Source: CAD feature listing. Evaluate the final solid. Frame: model axes, mm. Round coordinates to 2 decimals unless told otherwise and drop trailing zeros. Loops run counter-clockwise (first coordinate to the right, second up) from the corner with the lowest first, then second, coordinate; pieces in that order, holes last. Notation, with made-up numbers: M 25,42 L 39,42 A22 cw 39,54 Z; hole C -22.75,76.25 d9. An arc over 180 degrees is marked long. Answer as a JSON object with one key per item and string values.
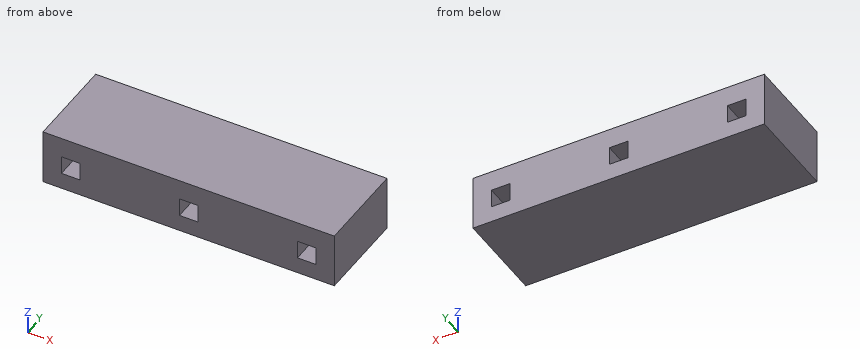
from build123d import *

# Parameters (mm, degrees)
SKETCH1_W           = 7.9
SKETCH1_H           = 1.5
SKETCH1_W_2         = 0.5
SKETCH1_H_2         = 0.5
BOSS_EXTRUDE1_DEPTH = 2.5


with BuildPart() as part:
    # Sketch1 → Boss-Extrude1 (new body)
    with BuildSketch(Plane(origin=(0, 0, 0), x_dir=(1, 0, 0), z_dir=(0, 1, 0))):
        with Locations((2.505127678, 0.264314746)):
            Rectangle(SKETCH1_W, SKETCH1_H)
        with Locations((-0.694872322, 0.316232633)):
            Rectangle(SKETCH1_W_2, SKETCH1_H_2, mode=Mode.SUBTRACT)
        with Locations((5.705127678, 0.319368521)):
            Rectangle(SKETCH1_W_2, SKETCH1_H_2, mode=Mode.SUBTRACT)
        with Locations((2.505127678, 0.311937798)):
            Rectangle(SKETCH1_W_2, SKETCH1_H_2, mode=Mode.SUBTRACT)
    extrude(amount=BOSS_EXTRUDE1_DEPTH)


solid = part.part
Item 1: Section B-B on y = 0.5. Return the cut outline in (x, z).
Answer sheet:
{"outline": "M -1.44,-1.01 L 6.46,-1.01 L 6.46,0.49 L -1.44,0.49 Z; hole M -0.94,-0.57 L -0.44,-0.57 L -0.44,-0.07 L -0.94,-0.07 Z; hole M 2.26,-0.56 L 2.76,-0.56 L 2.76,-0.06 L 2.26,-0.06 Z; hole M 5.46,-0.57 L 5.96,-0.57 L 5.96,-0.07 L 5.46,-0.07 Z"}
Item 2: Section A-A on x = 5.75. Return the cut outline in (y, z).
Answer sheet:
{"outline": "M 0,-1.01 L 2.5,-1.01 L 2.5,-0.57 L 0,-0.57 Z; M 0,-0.07 L 2.5,-0.07 L 2.5,0.49 L 0,0.49 Z"}
Item 3: Line query: probe 1 along X at (y, z) = (1.85, -0.5). Output: solid intervals per line, ascending. Write a range as from..to.
Answer sheet:
{"probe 1": "x = -1.44..-0.94, -0.44..2.26, 2.76..5.46, 5.96..6.46"}
Item 4: Section C-C on z = -0.3. Return the cut outline in (x, y), then the cut area to 3 significant figures.
Answer sheet:
{"outline": "M -1.44,0 L -0.94,0 L -0.94,2.5 L -1.44,2.5 Z; M -0.44,0 L 2.26,0 L 2.26,2.5 L -0.44,2.5 Z; M 2.76,0 L 5.46,0 L 5.46,2.5 L 2.76,2.5 Z; M 5.96,0 L 6.46,0 L 6.46,2.5 L 5.96,2.5 Z", "area": "16.0 mm²"}
